Build history of the part. All positions in model axes, mm. A direction names the side the tool comes from. Coordinates: 2 decimals unless noted, no trailing zeros. Order: outer loops, then holes, each group sorted by start corner. A loop starts at its lowest first (then second) coordinate and runs counter-clockwise, first axis right, second up. Notation, with made-up numbers: M 12,32.5 L 47,32.5 A23 cw 47,50.5 Z; hole C 68,-28.75 d11. An arc over 180 degrees is marked long. Write item = value, one per line. Start each with the question number.
Q1. Band-saw the part on B-B on z = 0. State how many separate pieces and enclosed holes the cut face has, plus the area to 3 significant figures.
Q2. Pin check, flat tips, straight feed: P1, Ø4, axis at x = 90, y = 7.5, coming from the -Z side; P2, Ø6.5, axis at x = 30, y = 7.5, coming from the +Z side; P3, Ø1.3, axis at y = 10, z = 10.5, coming from the +X side; P4, Ø3, axis at x = -93.5, y = 5.5, coming from the +Z side. Stop position of each tip, or through.
Q3. Band-saw the part on A-A on x = -115. Write the cut outline in (y, z), plus the area to 4 significant figures.
Q4. Pull direction Z, two halves, no side cores. Call faces 3 (the face through (-32.561, 8.306, 3.885)), 4 (the face through (-28, 6, -2)), 5 (the face through (143.4, 7.4, -0.1)), 6 (the face through (-136.6, 7.4, -0.1)): released by +Z, released by -Z, zero draft, split by the parting line, or undercut.
Q5. 3-axis set-ups, long thin cutter, end or side, ignore diameter. For faces 1 (the face through (-117.385, 7.395, -0.751)), 2 (the face through (-138, 7, 7.5)): which of +Z, -Z, +X, -X, +Y, -Y reach the whole face in a straight line?
Q6. Band-saw the part on D-D on x = 90. Write the cut outline in (y, z), plus the area to 3 significant figures.
Q7. Drill centre lines: probe 1 along Z at (x, y) = (-115, 5.75); probe 2 along Y at (x, z) = (90, 2.25); probe 3 along X at (y, z) = (3.25, -1). Where is each one in solid material? Low to high.
```python
from build123d import *

# Parameters (mm, degrees)
SKETCH_1_W                   = 300
SKETCH_1_H                   = 15
EXTRUDE_345_DEPTH            = 15
HOLE_WIZARD_M6_D             = 5
HOLE_WIZARD_M8_D             = 6.8
SKETCH_8_W                   = 250
SKETCH_8_H                   = 15
EXTRUDE_2518_DEPTH           = 5.4
SKETCH_10_W                  = 100
SKETCH_10_H                  = 15
CUT_EXTRUDE_2855_DEPTH       = 5.4
HOLE_WIZARD_1_M6_D           = 5
HOLE_WIZARD_1_M6_CSINK_D     = 12.6
HOLE_WIZARD_1_M6_CSINK_ANGLE = 90
HOLE_WIZARD_2_M6_D           = 5
HOLE_WIZARD_2_M6_CSINK_D     = 12.6
HOLE_WIZARD_2_M6_CSINK_ANGLE = 90
FILLET_1_R                   = 3
CHAMFER_1_SIZE               = 5
CHAMFER_2_SIZE               = 1


with BuildPart() as part:
    # Эскиз1 → Extrude 345 (new body)
    with BuildSketch(Plane(origin=(0, 0, 0), x_dir=(1, 0, 0), z_dir=(0, 1, 0))):
        Rectangle(SKETCH_1_W, SKETCH_1_H)
    extrude(amount=EXTRUDE_345_DEPTH)

    # Крепление шарнира M6 (through all)
    with Locations(Plane(origin=(0, 15, 0), x_dir=(1, 0, 0), z_dir=(0, 1, 0))):
        with Locations((-115, 0), (115, 0)):
            Hole(HOLE_WIZARD_M6_D / 2)

    # Шпилька-M8 (through all)
    with Locations(Plane(origin=(0, 15, 0), x_dir=(1, 0, 0), z_dir=(0, 1, 0))):
        with Locations((-140, 0), (140, 0)):
            Hole(HOLE_WIZARD_M8_D / 2)

    # Эскиз8 → Extrude 2518 (add)
    with BuildSketch(Plane.XY.offset(7.5)):
        with Locations((0, 7.5)):
            Rectangle(SKETCH_8_W, SKETCH_8_H)
    extrude(amount=EXTRUDE_2518_DEPTH)

    # Эскиз10 → Cut-Extrude 2855 (cut)
    with BuildSketch(Plane.XY.offset(12.9)):
        with Locations((0, 7.5)):
            Rectangle(SKETCH_10_W, SKETCH_10_H)
    extrude(amount=-CUT_EXTRUDE_2855_DEPTH, mode=Mode.SUBTRACT)

    # Прижим-1-M6 (through all)
    with Locations(Plane.XY.offset(12.9)):
        with Locations((-90, 7.5), (90, 7.5)):
            CounterSinkHole(HOLE_WIZARD_1_M6_D / 2, HOLE_WIZARD_1_M6_CSINK_D / 2, counter_sink_angle=HOLE_WIZARD_1_M6_CSINK_ANGLE)

    # Прижим-2-M6 (through all)
    with Locations(Plane.XY.offset(7.5)):
        with Locations((-30, 7.5), (30, 7.5)):
            CounterSinkHole(HOLE_WIZARD_2_M6_D / 2, HOLE_WIZARD_2_M6_CSINK_D / 2, counter_sink_angle=HOLE_WIZARD_2_M6_CSINK_ANGLE)

    # Скругление1
    fillet_1_edges = [part.edges().sort_by_distance(p)[0] for p in [
        (-50, 0, 10.2),
        (50, 0, 10.2),
    ]]
    fillet(fillet_1_edges, radius=FILLET_1_R)

    # Фаска1
    chamfer_1_edges = [part.edges().sort_by_distance(p)[0] for p in [
        (-150, 7.5, -7.5),
        (150, 7.5, -7.5),
    ]]
    chamfer(chamfer_1_edges, length=CHAMFER_1_SIZE)

    # Фаска2
    chamfer_2_edges = [part.edges().sort_by_distance(p)[0] for p in [
        (-125, 7.5, 12.9),
        (-89, 0, 12.9),
        (125, 7.5, 12.9),
        (-50, 9, 12.9),
        (50, 9, 12.9),
        (89, 0, 12.9),
        (50.878679656, 0.878679656, 12.9),
        (-50.878679656, 0.878679656, 12.9),
    ]]
    chamfer(chamfer_2_edges, length=CHAMFER_2_SIZE)


solid = part.part
```
Recorded:
q1.separate_pieces = 5
q1.enclosed_holes = 4
q1.area = 4,070 mm2
q2.P1 = through
q2.P2 = 4.45
q2.P3 = 125
q2.P4 = 12.13
q3.outline = M 0,-7.5 L 15,-7.5 L 15,-2.5 L 0,-2.5 Z; M 0,2.5 L 15,2.5 L 15,12.9 L 1,12.9 L 0,11.9 Z
q3.area = 230.5 mm2
q4.face_3 = released by +Z
q4.face_4 = zero draft
q4.face_5 = undercut
q4.face_6 = undercut
q5.face_1 = +Y, -Y
q5.face_2 = +Z, -X, +Y, -Y
q6.outline = M 0,-7.5 L 5,-7.5 L 5,9.1 L 1.2,12.9 L 1,12.9 L 0,11.9 Z; M 10,-7.5 L 15,-7.5 L 15,12.9 L 13.8,12.9 L 10,9.1 Z
q6.area = 189 mm2
q7.probe_1 = -7.5 to -2.5, 2.5 to 12.9
q7.probe_2 = 0 to 5, 10 to 15
q7.probe_3 = -150 to -143.25, -136.75 to -117.29, -112.71 to 112.71, 117.29 to 136.75, 143.25 to 150
